Autodesk Inventor part; units mm, degrees
ref_plane "YZ Plane" through (0, 0, 0) normal (1, 0, 0) x (0, 1, 0)
ref_plane "XZ Plane" through (0, 0, 0) normal (0, 1, 0) x (-1, 0, 0)
ref_plane "XY Plane" through (0, 0, 0) normal (0, 0, 1) x (1, 0, 0)
sketch "Sketch1" plane through (0, 0, 0) normal (0, 1, 0) x (-1, 0, 0)
  point P0 (0, 0)
sketch "Sketch2" plane through (0, 0, 0) normal (0, 1, 0) x (-1, 0, 0)
  line L0 (3.1195, 2.6996) -> (-11.8805, 2.6996)
  line L1 (-11.8805, 2.6996) -> (-11.8805, -2.3004)
  line L2 (-11.8805, -2.3004) -> (3.1195, -2.3004)
  line L3 (3.1195, -2.3004) -> (3.1195, 2.6996)
  point P0 (0, 0)
  dimension "d0" = 15
  dimension "d1" = 5
extrude "Extrusion1" add sketch "Sketch2" along normal blind 150
sketch "Sketch3" plane through (-3.1195, 0, 2.6996) normal (0, 0, 1) x (1, 0, 0)
  line L0 (15, 150) -> (0, 150)
  line L1 (15, 0) -> (15, 150)
  line L2 (0, 150) -> (15, 150)
  line L3 (15, 150) -> (15, 144.9614)
  line L4 (15, 144.9614) -> (0, 144.9614)
  line L5 (0, 144.9614) -> (0, 150)
  point P0 (3.1195, 0)
extrude "Extrusion2" add sketch "Sketch3" along normal blind 60
sketch "Sketch4" plane through (11.8805, 0, -2.3004) normal (0, 0, -1) x (-1, 0, 0)
  line L0 (0, 0) -> (15, 0)
  line L1 (0, 0) -> (15, 0)
  line L2 (15, 0) -> (15, 150)
  line L3 (0, 150) -> (15, 150)
  line L4 (0, 0) -> (0, 150)
  point P0 (11.8805, 0)
sketch "Sketch5" plane through (11.8805, 0, -2.3004) normal (0, 0, -1) x (-1, 0, 0)
  circle A0 centre (7.5, 10) radius 3 construction
  point P0 (11.8805, 0)
  dimension "d6" = 6
hole "Hole1" at (4.3805, 10, -2.3004) direction (0, 0, 1) diameter 6 end through all
Here's how the part is built. I have some questions about the finished solid (model axes, mm). A direction names the side the tool comes from. Coordinates: 2 decimals unless noted, no trailing zeros. Write each loop counter-clockwise with the first axis right and the second up, starting at its lowest first coordinate (ties: lowest second). Pieces come first, ordered by that corner, then holes. Notation, with made-up numbers: (26.5, 45.25) -> (72.5, 45.25) arc R21 cw to (72.5, 71.25) -> close; hole circle Ø8 at (-12, -35.5). An arc over 180 degrees is marked (long way). Use a Markdown table: item, result. Add a question column.
(1) We'd pull the mould along Y, two halves only. Please class faces 1 (the flat face through (4, 71, 2.7)), 2 (the flat face through (4, 150, 31)), 3 (the cylindrical face through (5.53, 12.77, 0.23)): +Y half, -Y half, draft (parallel to the pull), parting line (faces both ways), or undercut.
(2) I'm going to push flat-ended pins straight in: P1, Ø1.5, axis at x = -1.5, y = 38, coming from the +Z side; P2, Ø5, axis at x = 1.5, z = 35, coming from the -Y side. Where does each tip first touch, or does it pass through?
(3) If we section it at B-B, the plane x = 8.75: Write out the boundary of the cut face in (y, z), and give its area (3 significant figures).
(4) If we section it at A-A, the plane y = 10: Write out the boundary of the cut face in (x, z).
(5) Please list where these lines run through material, in increasing order: line 1 (X direction, y = 10, z = 0.95); line 2 (Y direction, x = -2.5, z = 18); line 3 (Z direction, x = -2, y = 29.5).
(6) If we section it at C-C, the plane z = 49: Write out the boundary of the cut face in (x, y).
(7) For faces 4 (the flat face through (4, 74, -2.3)), 5 (the flat face through (4, 144.961, 32)), which set-ups out of +Z, -Z, +X, -X, +Y, -Y let a thin tool reach every point of the face, with its end or its side?
(8) If we section it at D-D, the plane y = 72.5: Write out the boundary of the cut face in (x, z).
Outcome:
| question | item | result |
|---|---|---|
| 1 | face 1 | draft |
| 1 | face 2 | +Y half |
| 1 | face 3 | undercut |
| 2 | P1 | stops at z = 2.7 |
| 2 | P2 | stops at y = 144.96 |
| 3 | outline | (0, -2.3) -> (150, -2.3) -> (150, 62.7) -> (144.96, 62.7) -> (144.96, 2.7) -> (0, 2.7) -> close |
| 3 | area | 1,050 mm^2 |
| 4 | outline | (-3.12, -2.3) -> (1.38, -2.3) -> (1.38, 2.7) -> (-3.12, 2.7) -> close; (7.38, -2.3) -> (11.88, -2.3) -> (11.88, 2.7) -> (7.38, 2.7) -> close |
| 5 | line 1 | x = -3.12 to 1.38, 7.38 to 11.88 |
| 5 | line 2 | y = 144.96 to 150 |
| 5 | line 3 | z = -2.3 to 2.7 |
| 6 | outline | (-3.12, 144.96) -> (11.88, 144.96) -> (11.88, 150) -> (-3.12, 150) -> close |
| 7 | face 4 | -Z, +X, -X, +Y, -Y |
| 7 | face 5 | +Z, +X, -X, -Y |
| 8 | outline | (-3.12, -2.3) -> (11.88, -2.3) -> (11.88, 2.7) -> (-3.12, 2.7) -> close |
